Verification items for the finished model (mm, model axes). Coordinates: 2 decimals unless noted, no trailing zeros. Order: outer loops, then holes, each group sorted by start corner. A loop starts at its lowest first (then second) coordinate and runs counter-clockwise, first axis right, second up. Notation, with made-up numbers: M -34.75,-31.5 L -5.75,-31.5 A10 cw -5.75,-16.5 Z; hole C -11.75,51.5 d4. An arc over 180 degrees is marked long. Return JSON: item names as keys, results as strings. Group by question number.
1. Section check A-A, the plane x = 6. Record the cut outline in (y, z).
2. Gauge pin test, flat end, axial feed: pin 1 (6 mm diameter, centred on x = 6, y = 57, fed in from -Z). Record the tip position at first contact, or that the pin passes through.
3. Section check B-B, the plane y = 238. Record the cut outline in (x, z).
4. Material ranges on line 1 along Y through (x, z) = (6, 1.3); line 2 along X through (y, z) = (238, 1.2); line 3 along Y through (x, z) = (5, 2.8), recorded low to high.
```python
from build123d import *

# Parameters (mm, degrees)
SKETCH1_W                     = 12
SKETCH1_H                     = 245
PROFILE_DEPTH                 = 4
FASTENER_CLEARANCE_DEPTH      = 246.326313305
FASTENER_CLEARANCE_DEPTH_BACK = 246.326313305
SKETCH2_R                     = 2.25


with BuildPart() as part:
    # Sketch1 → Profile (new body)
    with BuildSketch(Plane.XY):
        with Locations((6, 122.5)):
            Rectangle(SKETCH1_W, SKETCH1_H)
    extrude(amount=PROFILE_DEPTH)

    # Sketch2 → Fastener_clearance (cut, two sides: drawn at the far end of the back side and taken through both)
    with BuildSketch(Plane.XY.offset(-FASTENER_CLEARANCE_DEPTH_BACK)):
        with Locations((6, 6)):
            Circle(SKETCH2_R)
        with Locations((6, 238)):
            Circle(SKETCH2_R)
    extrude(amount=FASTENER_CLEARANCE_DEPTH + FASTENER_CLEARANCE_DEPTH_BACK, mode=Mode.SUBTRACT)


solid = part.part
```
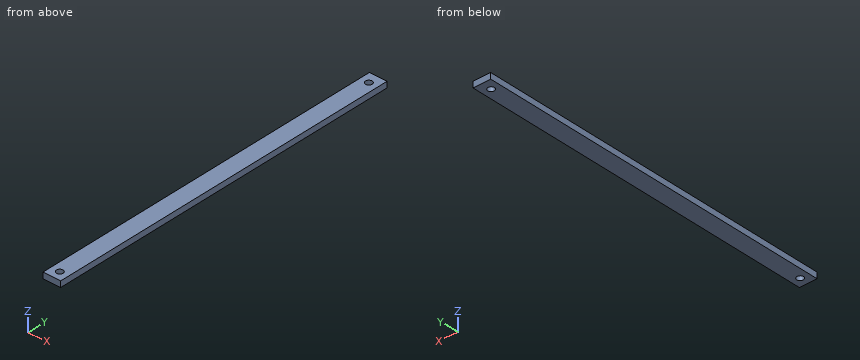
Answers follow:
{
 "1": {"outline": "M 0,0 L 3.75,0 L 3.75,4 L 0,4 Z; M 8.25,0 L 235.75,0 L 235.75,4 L 8.25,4 Z; M 240.25,0 L 245,0 L 245,4 L 240.25,4 Z"},
 "2": {"pin 1": "z = 0"},
 "3": {"outline": "M 0,0 L 3.75,0 L 3.75,4 L 0,4 Z; M 8.25,0 L 12,0 L 12,4 L 8.25,4 Z"},
 "4": {"line 1": "0 to 3.75, 8.25 to 235.75, 240.25 to 245", "line 2": "0 to 3.75, 8.25 to 12", "line 3": "0 to 3.98, 8.02 to 235.98, 240.02 to 245"}
}
